```python
from build123d import *

# Parameters (mm, degrees)
CASE_23X12P2X23_START                = -19
CASE_23X12P2X23_PROFILE_W            = 23
CASE_23X12P2X23_PROFILE_H            = 12.2
CASE_23X12P2X23_DEPTH                = 23
MOUNTING_EARS_33X12P2_START          = -2
MOUNTING_EARS_33X12P2_PROFILE_W      = 33
MOUNTING_EARS_33X12P2_PROFILE_H      = 12.2
MOUNTING_EARS_33X12P2_DEPTH          = 2
OUTPUT_ENVELOPE_NOT_SPLINE_START     = 4
OUTPUT_ENVELOPE_NOT_SPLINE_PROFILE_R = 2.5
OUTPUT_ENVELOPE_NOT_SPLINE_DEPTH     = 5


with BuildPart() as part:
    # Case_23x12p2x23_profile → Case_23x12p2x23 (new body)
    with BuildSketch(Plane.XY.offset(CASE_23X12P2X23_START)):
        with Locations((5.5, 0)):
            Rectangle(CASE_23X12P2X23_PROFILE_W, CASE_23X12P2X23_PROFILE_H)
    extrude(amount=CASE_23X12P2X23_DEPTH)

    # Mounting_ears_33x12p2_profile → Mounting_ears_33x12p2 (add)
    with BuildSketch(Plane.XY.offset(MOUNTING_EARS_33X12P2_START)):
        with Locations((5.5, 0)):
            Rectangle(MOUNTING_EARS_33X12P2_PROFILE_W, MOUNTING_EARS_33X12P2_PROFILE_H)
    extrude(amount=MOUNTING_EARS_33X12P2_DEPTH)

    # Output_envelope_not_spline_profile → Output_envelope_not_spline (add)
    with BuildSketch(Plane.XY.offset(OUTPUT_ENVELOPE_NOT_SPLINE_START)):
        Circle(OUTPUT_ENVELOPE_NOT_SPLINE_PROFILE_R)
    extrude(amount=OUTPUT_ENVELOPE_NOT_SPLINE_DEPTH)


solid = part.part
```
Can you work these out from the model? Positions are in its coordinate system, mm. A direction names the side the tool comes from. Coordinates: 2 decimals unless noted, no trailing zeros. Loops run counter-clockwise (first coordinate to the right, second up) from the corner with the lowest first, then second, coordinate; pieces in that order, holes last.
1) Imagine slicing it at B-B on x = 0. List the corners of the cut face in (y, z) for me.
2) Imagine slicing it at C-C on z = 5.25. List the corners of the cut face in (x, y) for me.
3) For pin 1 (3.5 mm diameter, centred on y = -1, z = -13, fed in from +X); pin 2 (1.5 mm diameter, centred on x = 19.5, y = 1, fed in from +Z); pin 3 (1.5 mm diameter, centred on x = 19.5, y = 2, fed in from -Z), each with a flat end and sliding along its axis, tell me the tip position at first contact or that it passes through.
4) Imagine slicing it at D-D on y = 0. List the corners of the cut face in (x, z) for me, plus the area to 3 significant figures.
5) Imagine slicing it at A-A on y = -4. List the corners of the cut face in (x, z) for me.
6) I need wall thicknesses on probe 1 along Z at (x, y) = (7, 3.75); probe 2 along Y at (x, z) = (0, 5); probe 3 along X at (y, z) = (2.75, -7). Which ranges of each line are inside material? Lowest first, please.
7) Which directions (+Z, -Z, +X, -X, +Y, -Y) give clear straight access to the entire face, cutting with the end or side of a thin tool? Please do faces 1 (the flat face through (19, 0, -2)), 2 (the flat face through (-9, 0, 0)), 3 (the cylindrical face through (-0.54, -2.44, 6.46)), 4 (the flat face through (-9, 0, -2)), 5 (the flat face through (17, 0, 2)).
Completed:
1. outline: (-6.1, -19) - (6.1, -19) - (6.1, 4) - (2.5, 4) - (2.5, 9) - (-2.5, 9) - (-2.5, 4) - (-6.1, 4) - close
2. outline: circle Ø5 at (0, 0)
3. pin 1: stops at x = 17
3. pin 2: stops at z = 0
3. pin 3: stops at z = -2
4. outline: (-11, -2) - (-6, -2) - (-6, -19) - (17, -19) - (17, -2) - (22, -2) - (22, 0) - (17, 0) - (17, 4) - (2.5, 4) - (2.5, 9) - (-2.5, 9) - (-2.5, 4) - (-6, 4) - (-6, 0) - (-11, 0) - close
4. area: 574 mm2
5. outline: (-11, -2) - (-6, -2) - (-6, -19) - (17, -19) - (17, -2) - (22, -2) - (22, 0) - (17, 0) - (17, 4) - (-6, 4) - (-6, 0) - (-11, 0) - close
6. probe 1: z = -19 to 4
6. probe 2: y = -2.5 to 2.5
6. probe 3: x = -6 to 17
7. face 1: -Z, +X, +Y, -Y
7. face 2: +Z, -X, +Y, -Y
7. face 3: +Z
7. face 4: -Z, -X, +Y, -Y
7. face 5: +Z, +X, +Y, -Y
